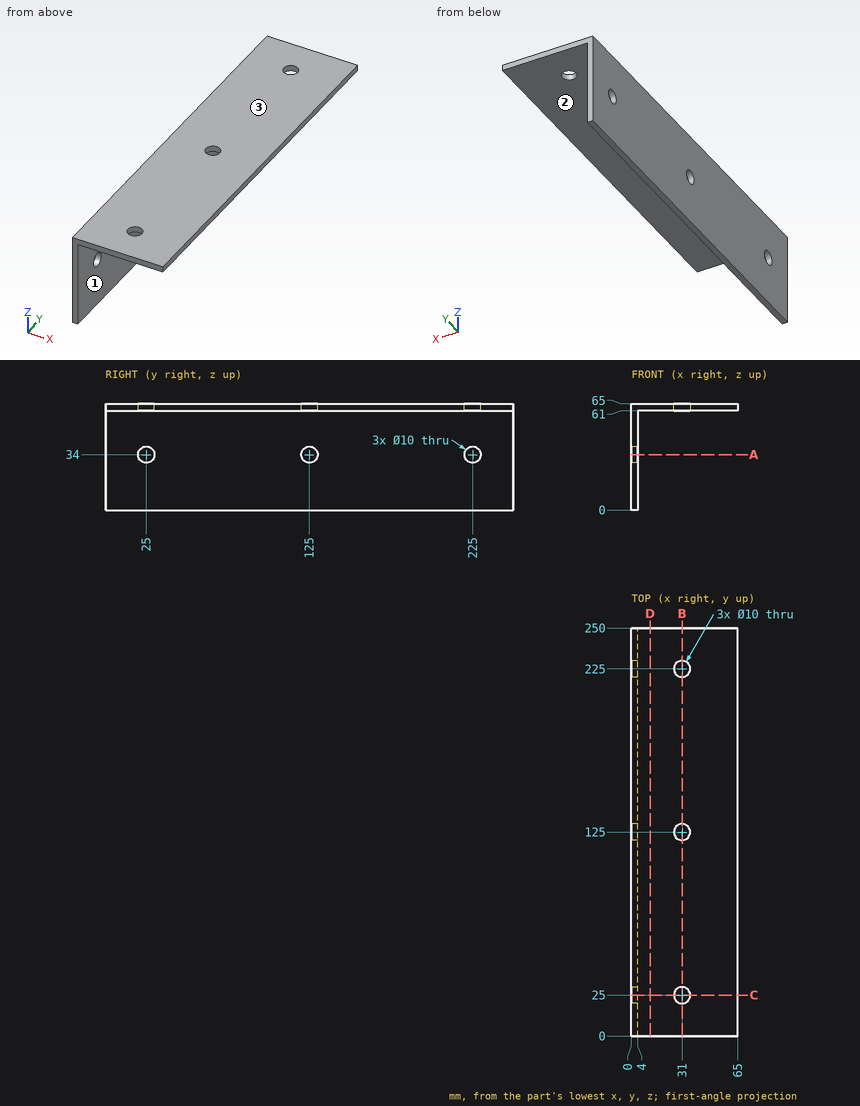
Study the drawing (mm; zero at the part's minimum x, y, z) and answer. Give positions to 0.01 mm unless a question says otherwise; leave off trailing zeros. Write each loop counter-clockwise with the first axis right and the second up, starting at its lowest first coordinate (ties: lowest second). Pieces come first, ordered by that corner, then holes. Notation, with made-up numbers: (43.25, -36) - (51.25, -36) arc R19 ccw to (51.25, -19) - close; hole circle Ø10 at (4.25, 49.5). An arc over 180 degrees is marked (long way). Use CSV: the item, a comma, the result in double quotes. Start each with the question number.
(1) Given P1, Ø1.5, axis at y = 50.5, z = 12, coming from the +X side; P2, Ø3, axis at x = 52.5, y = 147.5, coming from the -Z side, each flat-ended and moving along its own axis, determine where each tip first touches the part or whether it passes through.
(2) Consider line 1 along Y through (x, z) = (2, 34); line 2 along X through (y, z) = (29, 17); line 3 along Z through (x, y) = (49, 238.5). Determine where each line is inside the solid, lowest interval first.
(3) Find section D-D (x = 11.5). Give the vertices of the cut face in (y, z), plus the area to 3 significant figures.
(4) Find section C-C (y = 25). Give the vertices of the cut face in (x, z), plus the area to 3 significant figures.
(5) Find section B-B (x = 31). Give the vertices of the cut face in (y, z).
(6) Determine the mould class of the marked faces 1, 2 and 3 for opening direction Z: +Z half, -Z half, draft (parallel to the pull), parting line (faces both ways), or undercut.
(7) Find section A-A (z = 34). Give the vertices of the cut face in (x, y).
Findings below:
1,P1,"x = 4"
1,P2,"z = 61"
2,line 1,"0 to 20, 30 to 120, 130 to 220, 230 to 250"
2,line 2,"0 to 4"
2,line 3,"61 to 65"
3,outline,"(0, 61) - (250, 61) - (250, 65) - (0, 65) - close"
3,area,"1,000 mm2"
4,outline,"(0, 0) - (4, 0) - (4, 29) - (0, 29) - close; (0, 39) - (4, 39) - (4, 61) - (26, 61) - (26, 65) - (0, 65) - close; (36, 61) - (65, 61) - (65, 65) - (36, 65) - close"
4,area,"424 mm2"
5,outline,"(0, 61) - (20, 61) - (20, 65) - (0, 65) - close; (30, 61) - (120, 61) - (120, 65) - (30, 65) - close; (130, 61) - (220, 61) - (220, 65) - (130, 65) - close; (230, 61) - (250, 61) - (250, 65) - (230, 65) - close"
6,face 1,"draft"
6,face 2,"-Z half"
6,face 3,"+Z half"
7,outline,"(0, 0) - (4, 0) - (4, 20) - (0, 20) - close; (0, 30) - (4, 30) - (4, 120) - (0, 120) - close; (0, 130) - (4, 130) - (4, 220) - (0, 220) - close; (0, 230) - (4, 230) - (4, 250) - (0, 250) - close"
